Verification items for this drawing (mm, ordinates from the low corner). A direction names the side the tool comes from. Round coordinates to 2 decimals unless told otherwise and drop trailing zeros. Loops run counter-clockwise (first coordinate to the right, second up) from the corner with the lowest first, then second, coordinate; pieces in that order, holes last. Notation, with made-up numbers: (-7, 69.5) - (0, 69.5) arc R22 ccw to (0, 93.5) - close; hole circle Ø3 at (-33, 81). An arc over 180 degrees is marked (long way). Answer in a Markdown table with one row per item. Add a question column.
(1) Cross-section at C-C on y = 77.4. Enter the section's corners in (x, z).
(2) Mould release check, pull along X, two halves, no side actions. Record for the marked faces 1, 2 and 3: +X half, -X half, draft (parallel to the pull), parting line (faces both ways), or undercut.
(3) Cross-section at D-D on z = 24.5. Enter the section's corners in (x, y).
(4) Cross-section at B-B on x = 79. Enter the section's corners in (y, z), then the cut area to 3 significant figures.
(5) Thickness scan on line 1 along Y through (x, z) = (59, 1.4); line 2 along X through (y, z) = (71, 21); line 3 along Y through (x, z) = (55, 3). Record the ranges inside material, lowest first.
(6) Access from +Z, -Z, +X, -X, +Y, -Y to the whole of each face (thin tool, end or side, straight path). Record for the marked faces 4, 5 and 6.
(7) Gauge pin test, flat ends, axial feed: pin 1 (6 mm diameter, centred on y = 71, z = 24.5, fed in from +X); pin 2 (8 mm diameter, centred on x = 55, y = 7, fed in from +Z); pin 3 (8.5 mm diameter, centred on x = 59.5, z = 17, fed in from +Y). Record the tip position at first contact, or that the pin passes through.
(8) Cross-section at A-A on y = 7. Enter the section's corners in (x, z).
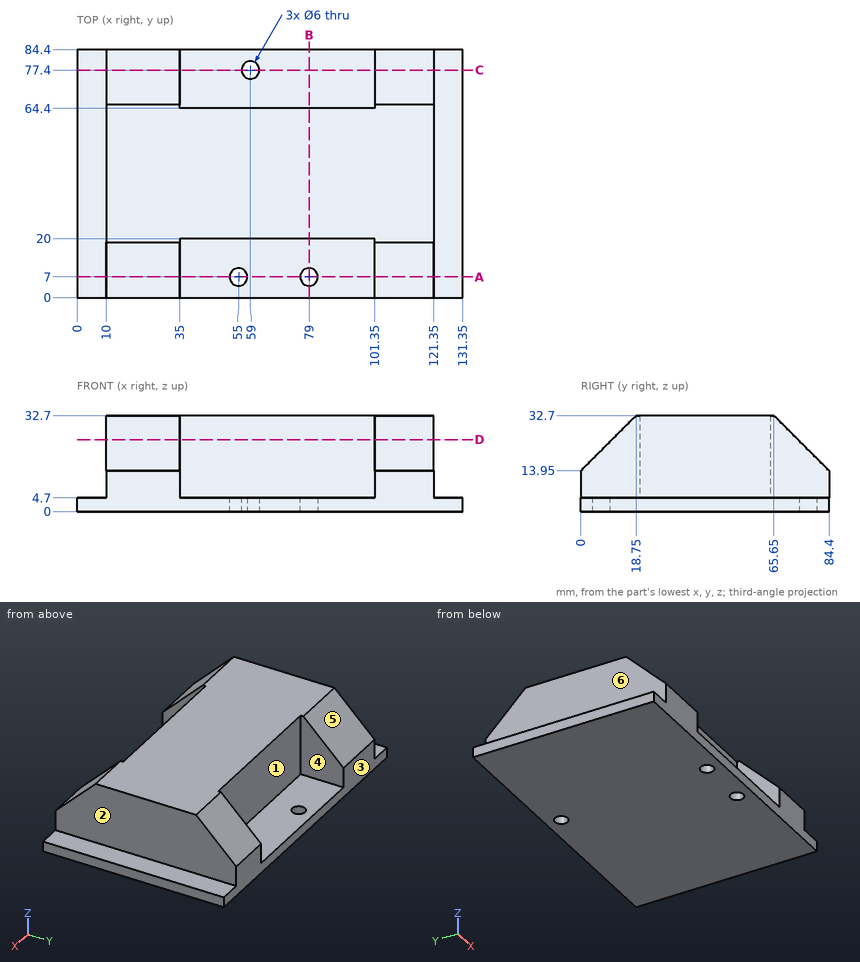
Answers:
| question | item | result |
|---|---|---|
| 1 | outline | (0, 0) - (56, 0) - (56, 4.7) - (35, 4.7) - (35, 20.95) - (10, 20.95) - (10, 4.7) - (0, 4.7) - close; (62, 0) - (131.35, 0) - (131.35, 4.7) - (121.35, 4.7) - (121.35, 20.95) - (101.35, 20.95) - (101.35, 4.7) - (62, 4.7) - close |
| 2 | face 1 | undercut |
| 2 | face 2 | +X half |
| 2 | face 3 | draft |
| 3 | outline | (10, 10.55) - (35, 10.55) - (35, 20) - (101.35, 20) - (101.35, 10.55) - (121.35, 10.55) - (121.35, 73.85) - (101.35, 73.85) - (101.35, 64.4) - (35, 64.4) - (35, 73.85) - (10, 73.85) - close |
| 4 | outline | (0, 0) - (4, 0) - (4, 4.7) - (0, 4.7) - close; (10, 0) - (84.4, 0) - (84.4, 4.7) - (64.4, 4.7) - (64.4, 32.7) - (20, 32.7) - (20, 4.7) - (10, 4.7) - close |
| 4 | area | 1,610 mm^2 |
| 5 | line 1 | y = 0 to 74.4, 80.4 to 84.4 |
| 5 | line 2 | x = 10 to 35, 101.35 to 121.35 |
| 5 | line 3 | y = 0 to 4, 10 to 84.4 |
| 6 | face 4 | +Z, +Y |
| 6 | face 5 | +Z, +X, -X, +Y |
| 6 | face 6 | +Z, -X, +Y, -Y |
| 7 | pin 1 | stops at x = 121.35 |
| 7 | pin 2 | stops at z = 4.7 |
| 7 | pin 3 | stops at y = 64.4 |
| 8 | outline | (0, 0) - (52, 0) - (52, 4.7) - (35, 4.7) - (35, 20.95) - (10, 20.95) - (10, 4.7) - (0, 4.7) - close; (58, 0) - (76, 0) - (76, 4.7) - (58, 4.7) - close; (82, 0) - (131.35, 0) - (131.35, 4.7) - (121.35, 4.7) - (121.35, 20.95) - (101.35, 20.95) - (101.35, 4.7) - (82, 4.7) - close |
